Could you check a few things on this model? Use its own coordinates, in mm. Face numbers are marked on the shaded views. Give positions to 0.01 mm unless a question says otherwise; leave off trailing zeros. Loops run counter-clockwise (first coordinate to the right, second up) from the corner with the lowest first, then second, coordinate; pieces in that order, holes last. Notation, with made-up numbers: (-28, 49.5) - (12, 49.5) arc R14 ccw to (12, 55.5) - close; hole circle Ø6 at (-15.5, 4). An arc over 180 degrees is marked (long way). Write each question's results on one line, items separated by ' | '. Start each with the question number.
1) I want a section at A-A, the plane x = 245. Write out the boundary of the cut face in (y, z) (3 decimals), and give its area (3 significant figures).
2) I want a section at D-D, the plane x = 88. Write out the boundary of the cut face in (y, z) (3 decimals), and give its area (3 significant figures).
3) I want a section at B-B, the plane y = 3.75. Write out the boundary of the cut face in (x, z) (3 decimals), and give its area (3 significant figures).
4) If we mould it in two halves opening along Z, with no side actions, what happens to the marked faces 1 and 2? For each: +Z half, -Z half, draft (parallel to the pull), parting line (faces both ways), or undercut.
5) If I drill on probe 1 along Z at (x, y) = (101.6, 23); probe 2 along Z at (x, y) = (255.27, 23.3) (3 decimals); probe 3 along Z at (x, y) = (182, 6) (3 decimals), over which ranges is the centre line in solid material (lowest first)? Write a range as [from, to].
6) I'm going to push flat-ended pins straight in: pin 1 (3 mm diameter, centred on x = 177.8, z = -254, fed in from -Y); pin 2 (2.5 mm diameter, centred on y = 23.5, z = -60, fed in from -X); pin 3 (6 mm diameter, centred on x = 171.5, z = -226, fed in from -Y) (3 decimals); pin 4 (1.6 mm diameter, centred on y = 23, z = -163.5, fed in from -X). Where does each tip first touch, or does it pass through?
7) I want a section at C-C, the plane z = -71. Write out the boundary of the cut face in (x, y) (3 decimals), and give its area (3 significant figures).
from build123d import *

# Parameters (mm, degrees)
SKETCH2_W           = 304.8
SKETCH2_H           = 266.7
BOSS_EXTRUDE1_DEPTH = 25.4
SKETCH12_W          = 260.35
SKETCH12_H          = 22.225
CUT_EXTRUDE8_DEPTH  = 305.8
CUT_EXTRUDE9_DEPTH  = 267.7
SKETCH14_R          = 14.2875
SKETCH14_R_2        = 3.175
CUT_EXTRUDE10_DEPTH = 4.175
CUT_EXTRUDE11_DEPTH = 3.175
SKETCH16_R          = 2.38125
CUT_EXTRUDE12_DEPTH = 267.7
SKETCH17_R          = 2.38125
CUT_EXTRUDE13_DEPTH = 26.4
SKETCH18_R          = 2.0955
CUT_EXTRUDE14_DEPTH = 3.175
SKETCH19_R          = 2.54
CUT_EXTRUDE15_DEPTH = 26.4
SKETCH20_R          = 2.54
CUT_EXTRUDE16_DEPTH = 26.4


with BuildPart() as part:
    # Sketch2 → Boss-Extrude1 (new body)
    with BuildSketch(Plane(origin=(0, 0, 0), x_dir=(1, 0, 0), z_dir=(0, 1, 0))):
        with Locations((152.4, 133.35)):
            Rectangle(SKETCH2_W, SKETCH2_H)
    extrude(amount=BOSS_EXTRUDE1_DEPTH)

    # Sketch12 → Cut-Extrude8 (cut, through all)
    with BuildSketch(Plane(origin=(304.8, 0, 0), x_dir=(0, 0, -1), z_dir=(1, 0, 0))):
        with Locations((133.35, 11.1125)):
            Rectangle(SKETCH12_W, SKETCH12_H)
    extrude(amount=-CUT_EXTRUDE8_DEPTH, mode=Mode.SUBTRACT)

    # Sketch13 → Cut-Extrude9 (cut, through all)
    with BuildSketch(Plane.XY):
        Polygon((304.8, 25.4), (279.4, 0), (304.8, 0), align=None)
        Polygon((0, 0), (0, 25.4), (25.4, 0), align=None)
    extrude(amount=-CUT_EXTRUDE9_DEPTH, mode=Mode.SUBTRACT)

    # Sketch14 → Cut-Extrude10 (cut, through all)
    with BuildSketch(Plane.XZ.offset(-22.225)):
        with Locations((18.415, -18.415)):
            Circle(SKETCH14_R)
        with Locations((18.415, -248.285)):
            Circle(SKETCH14_R)
        with Locations((255.27, -217.17)):
            Circle(SKETCH14_R_2)
    extrude(amount=-CUT_EXTRUDE10_DEPTH, mode=Mode.SUBTRACT)

    # Sketch15 → Cut-Extrude11 (cut)
    with BuildSketch(Plane(origin=(0, 25.4, 0), x_dir=(1, 0, 0), z_dir=(0, 1, 0))):
        with BuildLine():
            Line((44.45, 241.3), (139.7, 241.3))
            ThreePointArc((139.7, 241.3), (144.190128061, 239.440128061), (146.05, 234.95))
            Line((146.05, 234.95), (146.05, 152.4))
            ThreePointArc((146.05, 152.4), (144.190128061, 147.909871939), (139.7, 146.05))
            Line((139.7, 146.05), (44.45, 146.05))
            ThreePointArc((44.45, 146.05), (39.959871939, 147.909871939), (38.1, 152.4))
            Line((38.1, 152.4), (38.1, 234.95))
            ThreePointArc((38.1, 234.95), (39.959871939, 239.440128061), (44.45, 241.3))
        make_face()
        with BuildLine():
            Line((44.45, 120.65), (139.7, 120.65))
            ThreePointArc((139.7, 120.65), (144.190128061, 118.790128061), (146.05, 114.3))
            Line((146.05, 114.3), (146.05, 31.75))
            ThreePointArc((146.05, 31.75), (144.190128061, 27.259871939), (139.7, 25.4))
            Line((139.7, 25.4), (44.45, 25.4))
            ThreePointArc((44.45, 25.4), (39.959871939, 27.259871939), (38.1, 31.75))
            Line((38.1, 31.75), (38.1, 114.3))
            ThreePointArc((38.1, 114.3), (39.959871939, 118.790128061), (44.45, 120.65))
        make_face()
        with BuildLine():
            Line((177.8, 193.675), (273.05, 193.675))
            ThreePointArc((273.05, 193.675), (277.540128061, 191.815128061), (279.4, 187.325))
            Line((279.4, 187.325), (279.4, 152.4))
            ThreePointArc((279.4, 152.4), (277.540128061, 147.909871939), (273.05, 146.05))
            Line((273.05, 146.05), (177.8, 146.05))
            ThreePointArc((177.8, 146.05), (173.309871939, 147.909871939), (171.45, 152.4))
            Line((171.45, 152.4), (171.45, 187.325))
            ThreePointArc((171.45, 187.325), (173.309871939, 191.815128061), (177.8, 193.675))
        make_face()
        with BuildLine():
            Line((177.8, 120.65), (273.05, 120.65))
            ThreePointArc((273.05, 120.65), (277.540128061, 118.790128061), (279.4, 114.3))
            Line((279.4, 114.3), (279.4, 31.75))
            ThreePointArc((279.4, 31.75), (277.540128061, 27.259871939), (273.05, 25.4))
            Line((273.05, 25.4), (177.8, 25.4))
            ThreePointArc((177.8, 25.4), (173.309871939, 27.259871939), (171.45, 31.75))
            Line((171.45, 31.75), (171.45, 114.3))
            ThreePointArc((171.45, 114.3), (173.309871939, 118.790128061), (177.8, 120.65))
        make_face()
    extrude(amount=-CUT_EXTRUDE11_DEPTH, mode=Mode.SUBTRACT)

    # Sketch16 → Cut-Extrude12 (cut, through all)
    with BuildSketch(Plane.XY):
        with Locations((152.4, 12.7)):
            Circle(SKETCH16_R)
        with Locations((127, 12.7)):
            Circle(SKETCH16_R)
        with Locations((101.6, 12.7)):
            Circle(SKETCH16_R)
        with Locations((177.8, 12.7)):
            Circle(SKETCH16_R)
        with Locations((203.2, 12.7)):
            Circle(SKETCH16_R)
    extrude(amount=-CUT_EXTRUDE12_DEPTH, mode=Mode.SUBTRACT)

    # Sketch17 → Cut-Extrude13 (cut, through all)
    with BuildSketch(Plane(origin=(0, 25.4, 0), x_dir=(1, 0, 0), z_dir=(0, 1, 0))):
        with Locations((152.4, 12.7)):
            Circle(SKETCH17_R)
        with Locations((177.8, 12.7)):
            Circle(SKETCH17_R)
        with Locations((203.2, 12.7)):
            Circle(SKETCH17_R)
        with Locations((127, 12.7)):
            Circle(SKETCH17_R)
        with Locations((101.6, 12.7)):
            Circle(SKETCH17_R)
        with Locations((203.2, 254)):
            Circle(SKETCH17_R)
        with Locations((177.8, 254)):
            Circle(SKETCH17_R)
        with Locations((152.4, 254)):
            Circle(SKETCH17_R)
        with Locations((127, 254)):
            Circle(SKETCH17_R)
        with Locations((101.6, 254)):
            Circle(SKETCH17_R)
    extrude(amount=-CUT_EXTRUDE13_DEPTH, mode=Mode.SUBTRACT)

    # Sketch18 → Cut-Extrude14 (cut)
    with BuildSketch(Plane(origin=(0, 25.4, 0), x_dir=(1, 0, 0), z_dir=(0, 1, 0))):
        with Locations((255.27, 231.6734)):
            Circle(SKETCH18_R)
        with Locations((255.27, 202.6666)):
            Circle(SKETCH18_R)
    extrude(amount=-CUT_EXTRUDE14_DEPTH, mode=Mode.SUBTRACT)

    # Sketch19 → Cut-Extrude15 (cut, through all)
    with BuildSketch(Plane(origin=(0, 25.4, 0), x_dir=(1, 0, 0), z_dir=(0, 1, 0))):
        with Locations((196.85, 12.7)):
            Circle(SKETCH19_R)
    extrude(amount=-CUT_EXTRUDE15_DEPTH, mode=Mode.SUBTRACT)

    # Sketch20 → Cut-Extrude16 (cut, through all)
    with BuildSketch(Plane(origin=(0, 25.4, 0), x_dir=(1, 0, 0), z_dir=(0, 1, 0))):
        with Locations((292.1, 107.95)):
            Circle(SKETCH20_R)
    extrude(amount=-CUT_EXTRUDE16_DEPTH, mode=Mode.SUBTRACT)


solid = part.part
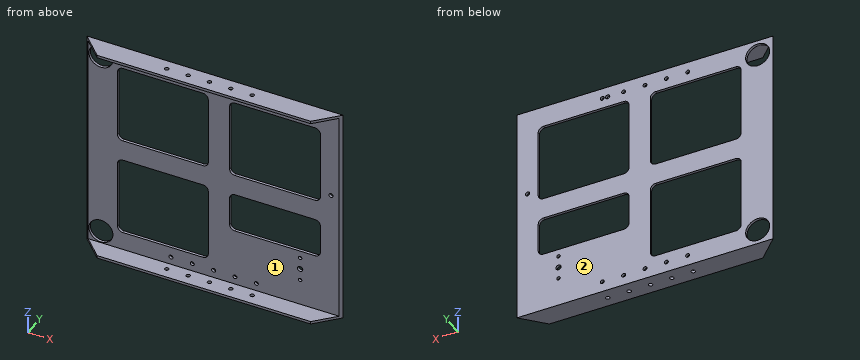
Answers:
1) outline: (0, -266.7) - (25.4, -266.7) - (25.4, -193.675) - (22.225, -193.675) - (22.225, -263.525) - (0, -263.525) - close; (0, -3.175) - (22.225, -3.175) - (22.225, -25.4) - (25.4, -25.4) - (25.4, 0) - (0, 0) - close; (22.225, -146.05) - (25.4, -146.05) - (25.4, -120.65) - (22.225, -120.65) - close | area: 534 mm2
2) outline: (0, -266.7) - (25.4, -266.7) - (25.4, -241.3) - (22.225, -241.3) - (22.225, -263.525) - (0, -263.525) - close; (0, -3.175) - (22.225, -3.175) - (22.225, -25.4) - (25.4, -25.4) - (25.4, 0) - (0, 0) - close; (22.225, -146.05) - (25.4, -146.05) - (25.4, -120.65) - (22.225, -120.65) - close | area: 383 mm2
3) outline: (21.65, -266.7) - (283.15, -266.7) - (283.15, -263.525) - (21.65, -263.525) - close; (21.65, -3.175) - (283.15, -3.175) - (283.15, 0) - (21.65, 0) - close | area: 1,660 mm2
4) face 1: undercut | face 2: draft
5) probe 1: z = [-266.7, -256.38], [-251.62, -241.3], [-146.05, -120.65], [-25.4, -15.08], [-10.32, 0] | probe 2: z = [-266.7, -233.769], [-229.578, -220.345], [-213.995, -204.762], [-200.571, -193.675], [-146.05, -120.65], [-25.4, 0] | probe 3: z = [-266.7, -263.525], [-3.175, 0]
6) pin 1: passes through | pin 2: stops at x = 0.65 | pin 3: stops at y = 22.225 | pin 4: stops at x = 1.6
7) outline: (0, 25.4) - (3.175, 22.225) - (38.1, 22.225) - (38.1, 25.4) - close; (146.05, 22.225) - (171.45, 22.225) - (171.45, 25.4) - (146.05, 25.4) - close; (279.4, 22.225) - (301.625, 22.225) - (304.8, 25.4) - (279.4, 25.4) - close | area: 272 mm2
